Geometry: final body of the model. Coordinates: model frame, mm. A direction names the side the tool comes from. Coordinates: 2 decimals unless noted, no trailing zeros. Write each loop counter-clockwise with the first axis right and the second up, starting at its lowest first coordinate (ties: lowest second). Pieces come first, ordered by that corner, then holes. Notation, with made-up numbers: (61.5, 48.5) - (78.5, 48.5) arc R24 cw to (78.5, 74.5) - close; hole circle Ø7 at (81.25, 38.25). An arc over 180 degrees is marked (long way). Answer as a JSON object with one key per item and string values. Group by question number.
Item 1: Line query: line 1 along Y through (x, z) = (-2.25, 4); line 2 along X through (y, z) = (2.5, 1.5); line 3 along Z through (x, y) = (-1, 1.25). Output: solid intervals per line, ascending. Write a range as from..to.
Item 2: Set-up query: faces 5 (the cylindrical face through (-0.69, 12.36, -3.1)), 6 (the flat face through (0.47, 1.88, -2.15)). Return all of +Z, -Z, +X, -X, +Y, -Y with unobstructed straight access to the full face (end or side cutting, diameter ignored); none if empty.
Item 3: Mould query, pull axis X, two halves, no side actions, for faces 1 (the flat face through (0, 3.81, 0)), 2 (the flat face through (2.095, 1.878, -0.672)), 3 (the flat face through (0, 19.05, 0)), 4 (the cylindrical face through (-3.78, 3.13, -2.9)). Classes: pulls with the +X half, pulls with the -X half, needs draft (parallel to the pull), parting line crosses it, or undercut.
Item 4: Section C-C on y = 13.5. Return loops of the section in (x, z) (3 decimals), and give its area (3 significant figures).
Item 5: First-contact query: pin 1 Ø1.5 at (x, z) = (1, 0.5) entering from -Y; pin 2 Ø1 at (y, z) = (11.5, -0.5) entering from +X (3 decimals); pin 3 Ø1 at (x, y) = (3, 5.5) entering from +Z. Flat tips, straight axial feed; report the tip coordinate or a pass-through.
Item 6: Section A-A on y = 1.25. Return loops of the section in (x, z) (1 decimal).
```python
from build123d import *

# Parameters (mm, degrees)
CHAMFER1_SIZE      = 0.508
CUT_EXTRUDE1_DEPTH = 3.81


with BuildPart() as part:
    # Sketch1 → Revolve1 (revolve)
    with BuildSketch(Plane.XY):
        Polygon((0, 0), (0, 19.05), (3.175, 19.05), (3.175, 6.35), (4.7625, 6.35), (4.7625, 0), align=None)
    revolve(axis=Axis((0, 19.05, 0), (0, -1, 0)))

    # Chamfer1
    chamfer1_edges = [part.edges().sort_by_distance(p)[0] for p in [
        (-3.175, 19.05, 0),
    ]]
    chamfer(chamfer1_edges, length=CHAMFER1_SIZE)

    # Sketch2 → Cut-Extrude1 (cut)
    with BuildSketch(Plane.XZ):
        Polygon((1.721936672, -1.867226311), (2.478033756, 0.557627746), (0.756097084, 2.424854057), (-1.721936672, 1.867226311), (-2.478033756, -0.557627746), (-0.756097084, -2.424854057), align=None)
    extrude(amount=-CUT_EXTRUDE1_DEPTH, mode=Mode.SUBTRACT)


solid = part.part
```
Checks:
{
 "1": {"line 1": "0..6.35", "line 2": "-4.52..-1.84, 1.61..4.52", "line 3": "-4.66..-2.16, 2.03..4.66"},
 "2": {"face 5": "+Y", "face 6": "-Y"},
 "3": {"face 1": "undercut", "face 2": "undercut", "face 3": "needs draft", "face 4": "parting line crosses it"},
 "4": {"outline": "circle Ø6.35 at (0, 0)", "area": "31.7 mm^2"},
 "5": {"pin 1": "y = 3.81", "pin 2": "x = 3.175", "pin 3": "z = 4.05"},
 "6": {"outline": "circle Ø9.5 at (0, 0); hole (-2.5, -0.6) - (-0.8, -2.4) - (1.7, -1.9) - (2.5, 0.6) - (0.8, 2.4) - (-1.7, 1.9) - close"}
}
